For this review, take the finished solid that the model builds, in its own axes (mm). A direction names the side the tool comes from. Give positions to 0.01 mm unless a question says otherwise; leave off trailing zeros. Write each loop counter-clockwise with the first axis right and the second up, starting at its lowest first coordinate (ties: lowest second). Pieces come first, ordered by that corner, then holes. Notation, with made-up numbers: (-23, 11) -> (9, 11) arc R23 ccw to (9, 27) -> close; hole circle Ø6 at (-18.5, -2). An arc over 180 degrees is marked (long way). Write item = value, one per line.
```python
from build123d import *

# Parameters (mm, degrees)
PAD_DEPTH    = 52
CHAMFER_SIZE = 2
FILLET_R     = 4


with BuildPart() as part:
    # Sketch → Pad (new body)
    with BuildSketch(Plane.XY):
        Polygon((0, 0), (75, 0), (75, -31), (46, -31), (46, -52), (75, -52), (75, -66), (0, -66), align=None)
    extrude(amount=PAD_DEPTH)

    # Chamfer
    chamfer_edges = [part.edges().sort_by_distance(p)[0] for p in [
        (37.5, 0, 0),
        (75, -15.5, 0),
        (60.5, -31, 0),
        (46, -41.5, 0),
        (60.5, -52, 0),
        (75, -59, 0),
        (37.5, -66, 0),
        (0, -33, 0),
    ]]
    chamfer(chamfer_edges, length=CHAMFER_SIZE)

    # Fillet
    fillet_edges = [part.edges().sort_by_distance(p)[0] for p in [
        (0, -66, 27),
        (75, -66, 27),
        (75, -52, 27),
        (75, -31, 27),
        (75, 0, 27),
        (46, -52, 27),
        (46, -31, 27),
        (0, 0, 27),
    ]]
    fillet(fillet_edges, radius=FILLET_R)


solid = part.part
```
(1) Take a section at C-C (y = -46.5). Write out the cut boundary in (x, z).
Answers below:
outline = (0, 2) -> (2, 0) -> (44, 0) -> (46, 2) -> (46, 52) -> (0, 52) -> close
(2) Take a section at D-D (x = 48.5). Write out the cut boundary in (y, z), plus the area to 3 significant figures.
Answers below:
outline = (-66, 2) -> (-64, 0) -> (-54, 0) -> (-51.71, 2.29) -> (-51.71, 52) -> (-66, 52) -> close; (-31.29, 2.29) -> (-29, 0) -> (-2, 0) -> (0, 2) -> (0, 52) -> (-31.29, 52) -> close
area = 2,360 mm^2
(3) To check wall thickness, follow probe 1 along Y at (x, z) = (67, 2.5); probe 2 along Y at (x, z) = (72, 18.5); probe 3 along X at (y, z) = (-39, 13). State the ranges of each line that lie inside material, in increasing order.
Answers below:
probe_1 = -66 to -52, -31 to 0
probe_2 = -65.87 to -52.13, -30.87 to -0.13
probe_3 = 0 to 46
(4) For pin 1 (12 mm diameter, centred on y = -35.5, z = 27.5, fed in from +X); pin 2 (6.5 mm diameter, centred on y = -41.5, z = 26.5, fed in from +X), all flat-tipped, find the tip position at first contact; note any pin that passes through.
Answers below:
pin_1 = 74.12
pin_2 = 46
(5) The part is to be moulded in two halves that separate along Y. For faces 1 (the face through (73.797, -64.859, 26.772)), 2 (the face through (37, 0, 27)), 3 (the face through (38, -33, 52)), 4 (the face through (61, -31, 27)), say which applies: released by +Y, released by -Y, zero draft, split by the parting line, or undercut.
Answers below:
face_1 = released by -Y
face_2 = released by +Y
face_3 = zero draft
face_4 = undercut
(6) Tool access review of faces 5 (the face through (59, -30, 1)), 6 (the face through (74, -59, 1)), 7 (the face through (73.859, -29.797, 26.772)): name each direction out of +Z, -Z, +X, -X, +Y, -Y from which nothing blocks a thin tool from reaching the whole face with its end or side.
Answers below:
face_5 = -Z, +X
face_6 = -Z, +X, +Y, -Y
face_7 = +Z, -Z, +X
(7) Take a section at A-A (x = 62.5). Write out the cut boundary in (y, z), plus the area to 3 significant figures.
Answers below:
outline = (-66, 2) -> (-64, 0) -> (-54, 0) -> (-52, 2) -> (-52, 52) -> (-66, 52) -> close; (-31, 2) -> (-29, 0) -> (-2, 0) -> (0, 2) -> (0, 52) -> (-31, 52) -> close
area = 2,330 mm^2
(8) Take a section at B-B (z = 42). Write out the cut boundary in (x, y).
Answers below:
outline = (0, -62) arc R4 ccw to (4, -66) -> (71, -66) arc R4 ccw to (75, -62) -> (75, -56) arc R4 ccw to (71, -52) -> (50, -52) arc R4 cw to (46, -48) -> (46, -35) arc R4 cw to (50, -31) -> (71, -31) arc R4 ccw to (75, -27) -> (75, -4) arc R4 ccw to (71, 0) -> (4, 0) arc R4 ccw to (0, -4) -> close
